Input: dimensioned drawing with shaded views. Units: mm. Origin: part minimum x, y, z. Give positions to 0.01 mm unless a question says otherwise; leave off trailing zeros. Loops run counter-clockwise (first coordinate to the right, second up) from the corner with the lowest first, then second, coordinate; pieces in that order, holes last. Notation, with made-up numbers: M -33,72 L 21,72 A14 ccw 21,83 Z; hole C -30,4.25 d6. An arc over 180 degrees is marked long. Use CSV: the item, a comma, the result in double quotes. Start each with the question number.
Q1. Pin query (flat end, axial travel): pin 1 (4.5 mm diameter, centred on x = 190.5, y = 6.5, fed in from -Z); pin 2 (23 mm diameter, centred on x = 25, z = 475, fed in from -Y). Return the tip coordinate at first contact, or that it passes through.
Q2. Material intervals for line 1 along Z through (x, y) = (71.5, 2.5) (3 decimals); line 2 along X through (y, z) = (10.25, 475); line 3 along X through (y, z) = (11.5, 341), sorted ascending.
Q3. Section C-C, the plane y = 11.75. Output: boundary loops of the cut face in (x, z) (3 decimals).
Q4. Section B-B, the plane z = 379.5. Output: boundary loops of the cut face in (x, y), plus the area to 3 significant figures.
Q5. Section A-A, the plane x = 243. Output: boundary loops of the cut face in (y, z) (3 decimals), plus the area to 3 significant figures.
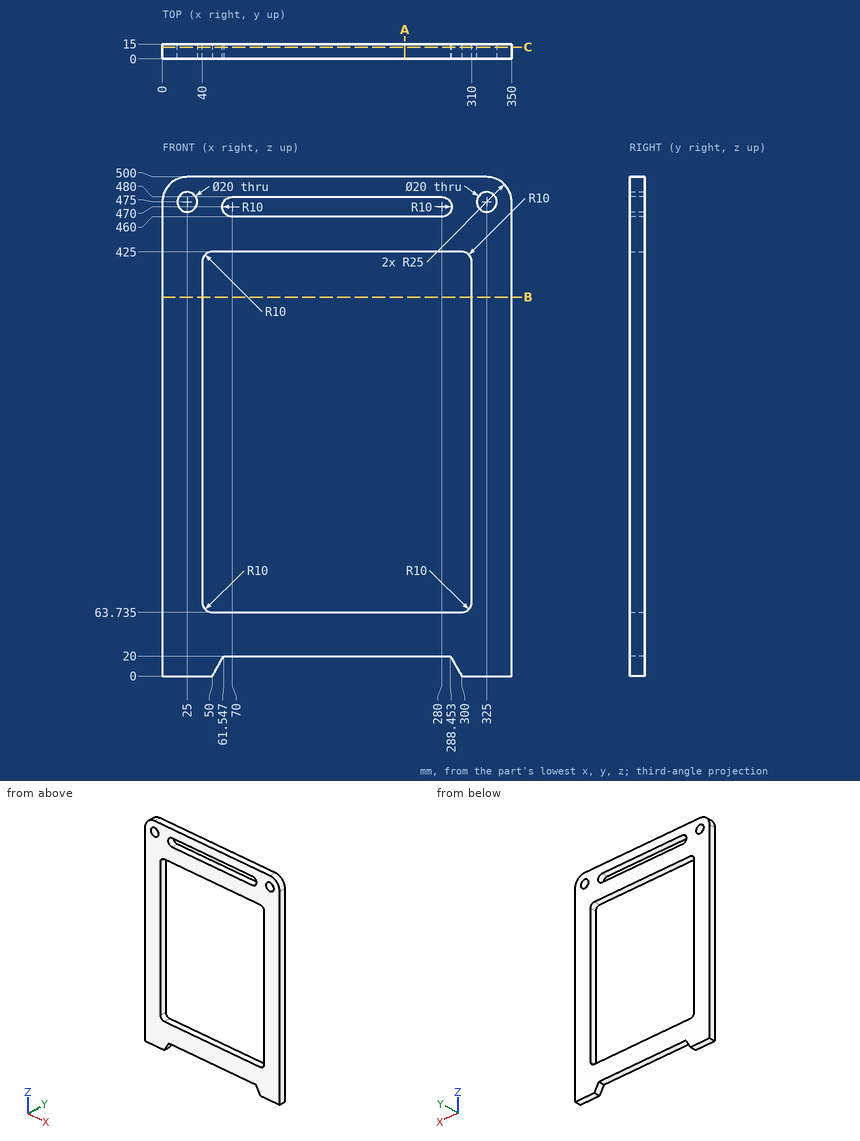
A:
1,pin 1,"z = 20"
1,pin 2,"y = 0"
2,line 1,"20 to 63.735, 425 to 460, 480 to 500"
2,line 2,"0 to 15, 35 to 61.34, 288.66 to 315, 335 to 350"
2,line 3,"0 to 40, 310 to 350"
3,outline,"M 0,0 L 50,0 L 61.547,20 L 288.453,20 L 300,0 L 350,0 L 350,475 A25 ccw 325,500 L 25,500 A25 ccw 0,475 Z; hole C 25,475 d20; hole M 40,73.735 A10 ccw 50,63.735 L 300,63.735 A10 ccw 310,73.735 L 310,415 A10 ccw 300,425 L 50,425 A10 ccw 40,415 Z; hole M 70,460 L 280,460 A10 ccw 280,480 L 70,480 A10 ccw Z; hole C 325,475 d20"
4,outline,"M 0,0 L 40,0 L 40,15 L 0,15 Z; M 310,0 L 350,0 L 350,15 L 310,15 Z"
4,area,"1,200 mm^2"
5,outline,"M 0,20 L 15,20 L 15,63.735 L 0,63.735 Z; M 0,425 L 15,425 L 15,460 L 0,460 Z; M 0,480 L 15,480 L 15,500 L 0,500 Z"
5,area,"1,480 mm^2"
